Autodesk Fusion 360 part; units mm, degrees
sketch "Sketch1" plane through (0, 0, 0) normal (0, 0, 1) x (1, 0, 0) in component "Mount"
  line L0 (20, 14) -> (-20, 14)
  line L1 (-20, 14) -> (-20, -14)
  line L2 (-20, -14) -> (20, -14)
  line L3 (20, -14) -> (20, 14)
  line L4 (20, 14) -> (-20, -14) construction
  line L5 (-20, 14) -> (20, -14) construction
  dimension "d1" = 40
  dimension "d2" = 28
extrude "Extrude1" add sketch "Sketch1" along normal blind 24 in component "Mount"
sketch "Sketch2" plane through (0, 0, 24) normal (0, 0, 1) x (-1, 0, 0) in component "Mount"
  line L0 (-20, 14) -> (-20, -14)
  line L1 (-20, -14) -> (20, -14)
  line L2 (20, -14) -> (20, 14)
  line L3 (20, 14) -> (-20, 14)
  line L4 (20, -10) -> (0, -10)
  line L5 (0, -10) -> (0, 10)
  line L6 (0, 10) -> (20, 10)
  line L7 (20, 10) -> (20, -10)
  dimension "d5" = 20
  dimension "d6" = 20
  dimension "d7" = 4
extrude "Extrude2" cut sketch "Sketch2" against normal blind 20 contours L2 L4 L5 L6 L7 in component "Mount"
sketch "Sketch3" plane through (0, -14, 0) normal (0, -1, 0) x (1, 0, 0) in component "Mount"
  line L0 (-20, 0) -> (20, 0)
  line L1 (20, 0) -> (20, 24)
  line L2 (20, 24) -> (-20, 24)
  line L3 (-20, 24) -> (-20, 0)
  line L4 (-8, 0) -> (-8, 24) construction
  line L5 (-20, 14) -> (20, 14) construction
  circle A0 centre (-8, 14) radius 2.5
  circle A1 centre (-8, 14) radius 4.5
  dimension "d10" = 12
  dimension "d11" = 10
  dimension "d12" = 5
  dimension "d13" = 9
extrude "Extrude4" cut sketch "Sketch3" against normal blind 1 contours A0 | A1 in component "Mount"
extrude "Extrude3" cut sketch "Sketch3" against normal blind 4 contours A0 in component "Mount"
sketch "Sketch4" plane through (0, 14, 0) normal (0, 1, 0) x (-1, 0, 0) in component "Mount"
  line L0 (-20, 0) -> (20, 0)
  line L1 (20, 0) -> (20, 24)
  line L2 (20, 24) -> (-20, 24)
  line L3 (-20, 24) -> (-20, 0)
  line L4 (14, 24) -> (14, 0) construction
  line L5 (20, 14) -> (-20, 14) construction
  circle A0 centre (14, 14) radius 2.5
  circle A1 centre (14, 14) radius 4.5
  dimension "d18" = 10
  dimension "d19" = 6
  dimension "d20" = 5
  dimension "d21" = 9
extrude "Extrude6" cut sketch "Sketch4" against normal blind 1 contours A0 | A1 in component "Mount"
extrude "Extrude5" cut sketch "Sketch4" against normal blind 4 contours A0 in component "Mount"
sketch "Sketch5" plane through (0, 0, 24) normal (0, 0, 1) x (-1, 0, 0) in component "Mount"
  line L0 (0, 10) -> (20, 10)
  line L1 (20, 10) -> (20, 14)
  line L2 (20, 14) -> (-20, 14)
  line L3 (-20, 14) -> (-20, -14)
  line L4 (-20, -14) -> (20, -14)
  line L5 (20, -14) -> (20, -10)
  line L6 (20, -10) -> (0, -10)
  line L7 (0, -10) -> (0, 10)
  line L8 (0, -10) -> (-20, -10) construction
  line L9 (0, 10) -> (-20, 10) construction
  line L10 (-20, 10) -> (0, -10) construction
  line L11 (0, 10) -> (-20, -10) construction
  circle A0 centre (-10, 0) radius 8
  circle A1 centre (-10, 0) radius 4
  circle A2 centre (-10, 0) radius 2
  dimension "d26" = 16
  dimension "d27" = 8
  dimension "d28" = 4
extrude "Extrude7" cut sketch "Sketch5" against normal blind 6 contours A0 | A1 | A2 in component "Mount"
extrude "Extrude8" add sketch "Sketch5" along normal blind 4 from surface at -6 contours A1 in component "Mount"
extrude "Extrude9" cut sketch "Sketch5" against normal blind 18.3 contours A2 in component "Mount"
fillet "Fillet2" radius 2 4 edges at (20, 14, 12) (20, -14, 12) (-20, -14, 12) (-20, 14, 12) in component "Mount"
sketch "Sketch6" plane through (0, 0, 0) normal (0, 0, -1) x (1, 0, 0) in component "Mount"
  arc A0 (-20, -12) -> (-18, -14) centre (-18, -12) ccw
  line L0 (-18, -14) -> (18, -14)
  arc A1 (18, -14) -> (20, -12) centre (18, -12) ccw
  line L1 (20, -12) -> (20, 12)
  arc A2 (20, 12) -> (18, 14) centre (18, 12) ccw
  line L2 (18, 14) -> (-18, 14)
  arc A3 (-18, 14) -> (-20, 12) centre (-18, 12) ccw
  line L3 (-20, 12) -> (-20, -12)
  line L4 (12.8, -1.6166) -> (12.8, 1.6166)
  line L5 (12.8, 1.6166) -> (10, 3.2332)
  line L6 (10, 3.2332) -> (7.2, 1.6166)
  line L7 (7.2, 1.6166) -> (7.2, -1.6166)
  line L8 (7.2, -1.6166) -> (10, -3.2332)
  line L9 (10, -3.2332) -> (12.8, -1.6166)
  line L10 (10, 0) -> (10, 14) construction
  point P0 (10, 0)
  dimension "d50" = 2.8
extrude "Extrude10" cut sketch "Sketch6" against normal blind 5.5 contours L4 L5 L6 L7 L8 L9 in component "Mount"
component "Mount" placed x (1, 0, 0) y (0, 1, 0) z (0, 0, 1) at (0, 0, 0)
properties part number "Mount"
Model file for the job. Use its own axes, mm. A direction names the side the tool comes from. Round coordinates to 2 decimals unless told otherwise and drop trailing zeros. Loops run counter-clockwise (first coordinate to the right, second up) from the corner with the lowest first, then second, coordinate; pieces in that order, holes last. Notation, with made-up numbers: (51, 88.25) -> (108, 88.25) arc R22 cw to (108, 109.25) -> close; hole circle Ø7 at (-20, 48). An arc over 180 degrees is marked (long way). Answer as CSV lines item,"result". Start each with the question number.
1) Slice it at C-C (z = 10.5). List the corners of the cut face in (x, y).
2) Pin check, flat tips, straight feed: P1, Ø1, axis at x = -6, z = 16, coming from the -Y side; P2, Ø7, axis at x = -16, z = 13, coming from the +Y side; P3, Ø6, axis at x = -8.5, y = 1.5, coming from the +Z side; P4, Ø4.5, axis at x = 9.5, y = -0.5, coming from the +Z side. Stop position of each tip, or through.
3) Tool access for faces 5 (the face through (12.8, 0, 3)), 6 (the face through (11.73, 7.81, 21.04)), 7 (the face through (0, 0, 14)): list every direction of +Z, -Z, +X, -X, +Y, -Y with a clear straight run to the whole face (end or side of a thin tool).
4) Slice it at A-A (x = -3). List the corners of the cut face in (y, z).
5) Slice it at D-D (y = 0). List the corners of the cut face in (x, z), plus the area to 3 significant figures.
6) Mould opens along Z. For faces 1 (the face through (0, -14, 12)), 2 (the face through (8, -4, 18)), 3 (the face through (-5.581, -13.507, 17.794)), 4 (the face through (-16, 13, 12)) say: +Z half, -Z half, draft (parallel to the pull), parting line (faces both ways), or undercut.
7) Slice it at B-B (x = -14). List the corners of the cut face in (y, z), plus the area to 3 significant figures.
8) Probe line 1 along Z through (x, y) = (-14, 13.3); line 2 along Y through (x, z) = (-3.5, 9.5); line 3 along X through (y, z) = (0, 20.5). List the from-to ranges inside material, lowest first.
Filled in:
1,outline,"(-20, -12) arc R2 ccw to (-18, -14) -> (-10.83, -14) -> (-10.83, -13) -> (-5.17, -13) -> (-5.17, -14) -> (18, -14) arc R2 ccw to (20, -12) -> (20, 12) arc R2 ccw to (18, 14) -> (-11.17, 14) -> (-11.17, 13) -> (-16.83, 13) -> (-16.83, 14) -> (-18, 14) arc R2 ccw to (-20, 12) -> (-20, 10) -> (0, 10) -> (0, -10) -> (-20, -10) -> close; hole circle Ø4 at (10, 0)"
2,P1,"stops at y = -13"
2,P2,"stops at y = 14"
2,P3,"stops at z = 4"
2,P4,"stops at z = 22"
3,face 5,"-Z"
3,face 6,"+Z"
3,face 7,"+Z, -X"
4,outline,"(-14, 0) -> (14, 0) -> (14, 24) -> (10, 24) -> (10, 4) -> (-10, 4) -> (-10, 24) -> (-14, 24) -> close"
5,outline,"(-20, 0) -> (7.2, 0) -> (7.2, 5.5) -> (12.8, 5.5) -> (12.8, 0) -> (20, 0) -> (20, 24) -> (18, 24) -> (18, 18) -> (14, 18) -> (14, 22) -> (12, 22) -> (12, 5.7) -> (8, 5.7) -> (8, 22) -> (6, 22) -> (6, 18) -> (2, 18) -> (2, 24) -> (0, 24) -> (0, 4) -> (-20, 4) -> close"
5,area,"400 mm2"
6,face 1,"draft"
6,face 2,"+Z half"
6,face 3,"undercut"
6,face 4,"undercut"
7,outline,"(-14, 0) -> (14, 0) -> (14, 9.5) -> (13, 9.5) -> (13, 11.5) -> (10, 11.5) -> (10, 4) -> (-10, 4) -> (-10, 24) -> (-14, 24) -> close; (10, 16.5) -> (13, 16.5) -> (13, 18.5) -> (14, 18.5) -> (14, 24) -> (10, 24) -> close"
7,area,"248 mm2"
8,line 1,"z = 0 to 9.5, 18.5 to 24"
8,line 2,"y = -14 to -10, 10 to 14"
8,line 3,"x = 0 to 2, 6 to 8, 12 to 14, 18 to 20"
